```python
from build123d import *

# Parameters (mm, degrees)
SKETCH_1_W                  = 300
SKETCH_1_H                  = 30
EXTRUDE_1_DEPTH             = 5
CHAMFER_1_SIZE              = 1
HOLE_WIZARD_M3_1_D          = 3.2
M3X0_5_1_D                  = 2.5
M4X0_7_1_D                  = 3.3
M4X0_7_2_D                  = 3.3
PATTERN_LINEAR_1_COUNT      = 6
PATTERN_LINEAR_1_PITCH      = 25
PATTERN_LINEAR_1_COL_COUNT  = 7
PATTERN_LINEAR_1_COL_PITCH  = 25
EXTRUDE_3_DEPTH             = 5
SKETCH_13_R                 = 6.1
CUT_EXTRUDE_2_DEPTH         = 161.542829177
HOLE_WIZARD_M2_1_D          = 2.2
M4X0_7_3_D                  = 3.3
HOLE_WIZARD_M4_1_D          = 4.3
M3X0_5_2_D                  = 2.5
CUT_EXTRUDE_3_DEPTH         = 161.542829177
CUT_EXTRUDE_3_DEPTH_BACK    = 161.542829177
SKETCH_25_W                 = 15
SKETCH_25_H                 = 5
FILLET_1_R                  = 1
SKETCH_26_W                 = 30
SKETCH_26_H                 = 5
EXTRUDE_4_DEPTH             = 30
SKETCH_27_R                 = 1.65
CUT_EXTRUDE_4_DEPTH         = 174.476223155
PATTERN_LINEAR_2_COUNT      = 2
PATTERN_LINEAR_2_PITCH      = 20
PATTERN_LINEAR_2_COUNT_DIR2 = 3
PATTERN_LINEAR_2_PITCH_DIR2 = 10
FILLET_2_R                  = 5
HOLE_WIZARD_M3_2_D          = 3.2


with BuildPart() as part:
    # 草圖1 → 填料-伸長1 (new body)
    with BuildSketch(Plane.XY):
        Rectangle(SKETCH_1_W, SKETCH_1_H)
    extrude(amount=EXTRUDE_1_DEPTH)

    # 導角1
    chamfer_1_edges = [part.edges().sort_by_distance(p)[0] for p in [
        (150, -15, 2.5),
        (-150, -15, 2.5),
        (-150, 15, 2.5),
        (150, 15, 2.5),
    ]]
    chamfer(chamfer_1_edges, length=CHAMFER_1_SIZE)

    # M3 餘隙孔1 (through all)
    with Locations(Plane.XY.offset(5)):
        with Locations((20, -10), (20, 10), (0, -10), (0, 10)):
            Hole(HOLE_WIZARD_M3_1_D / 2)

    # M3x0.5 螺紋孔1 (through all)
    with Locations(Plane.XY.offset(5)):
        with Locations((-12.5, 0)):
            m3x0_5_1 = Hole(M3X0_5_1_D / 2)

    # M4x0.7 螺紋孔1 (through all)
    with Locations(Plane.XY.offset(5)):
        with Locations((100, 10), (70, -10), (70, 10), (100, -10), (85, 10), (85, -10)):
            Hole(M4X0_7_1_D / 2)

    # M4x0.7 螺紋孔2 (through all)
    with Locations(Plane.XY.offset(5)):
        with Locations((-126, 10), (-126, -10)):
            m4x0_7_2 = Hole(M4X0_7_2_D / 2)

    # 直線複製排列1: M3x0.5 螺紋孔1 ×6
    with Locations(*[(-i * PATTERN_LINEAR_1_PITCH, 0, 0) for i in range(1, PATTERN_LINEAR_1_COUNT)]):
        add(m3x0_5_1, mode=Mode.SUBTRACT)

    # 直線複製排列1 col: M3x0.5 螺紋孔1 ×7
    with Locations(*[(i * PATTERN_LINEAR_1_COL_PITCH, 0, 0) for i in range(1, PATTERN_LINEAR_1_COL_COUNT)]):
        add(m3x0_5_1, mode=Mode.SUBTRACT)

    # 鏡射1: M4x0.7 螺紋孔2 across plane
    add(m4x0_7_2.mirror(Plane(origin=(0, 0, 0), x_dir=(0, 0, 1), z_dir=(1, 0, 0))), mode=Mode.SUBTRACT)

    # 草圖16 → 填料-伸長3 (add, through all)
    with BuildSketch(Plane.XY):
        with BuildLine():
            Line((-20, 15), (64, 15))
            Line((64, 15), (64, 57))
            Line((64, 57), (0, 57))
            ThreePointArc((0, 57), (-14.142135624, 51.142135624), (-20, 37))
            Line((-20, 37), (-20, 15))
        make_face()
    extrude(amount=EXTRUDE_3_DEPTH)

    # 草圖13 → 除料-伸長2 (cut, through all)
    with BuildSketch(Plane.XY):
        with Locations(Location((44, 24.8, 0), (0, 0, 180))):
            Circle(SKETCH_13_R)
    extrude(amount=CUT_EXTRUDE_2_DEPTH, mode=Mode.SUBTRACT)

    # M2 餘隙孔1 (through all)
    with Locations(Plane.XY.offset(5)):
        with Locations((39, 24.8), (49, 24.8)):
            Hole(HOLE_WIZARD_M2_1_D / 2)

    # M4x0.7 螺紋孔3 (through all)
    with Locations(Plane.XY.offset(5)):
        with Locations((15, 22), (-15, 22)):
            Hole(M4X0_7_3_D / 2)

    # M4 餘隙孔1 (through all)
    with Locations(Plane.XY.offset(5)):
        with Locations((-26, -10), (-26, 10), (-50, -10), (-50, 10)):
            Hole(HOLE_WIZARD_M4_1_D / 2)

    # M3x0.5 螺紋孔2 (through all)
    with Locations(Plane.XY.offset(5)):
        with Locations((33, 53), (33, 45)):
            Hole(M3X0_5_2_D / 2)

    # 草圖25 → 除料-伸長3 (cut, two sides: drawn at the far end of the back side and taken through both)
    with BuildSketch(Plane.XY.offset(5).offset(-CUT_EXTRUDE_3_DEPTH_BACK)):
        with Locations((33, 38.5)):
            Rectangle(SKETCH_25_W, SKETCH_25_H)
    extrude(amount=CUT_EXTRUDE_3_DEPTH + CUT_EXTRUDE_3_DEPTH_BACK, mode=Mode.SUBTRACT)

    # 圓角1
    fillet_1_edges = [part.edges().sort_by_distance(p)[0] for p in [
        (40.5, 41, 2.5),
        (40.5, 36, 2.5),
        (25.5, 36, 2.5),
        (25.5, 41, 2.5),
    ]]
    fillet(fillet_1_edges, radius=FILLET_1_R)

    # 草圖26 → 填料-伸長4 (add)
    with BuildSketch(Plane(origin=(0, 57, 0), x_dir=(1, 0, 0), z_dir=(0, 1, 0))):
        with Locations((35, -2.5)):
            Rectangle(SKETCH_26_W, SKETCH_26_H)
    extrude(amount=EXTRUDE_4_DEPTH)

    # 草圖27 → 除料-伸長4 (cut, through all)
    with BuildSketch(Plane.XY.offset(5)):
        with Locations((25, 82)):
            Circle(SKETCH_27_R)
    cut_extrude_4 = extrude(amount=-CUT_EXTRUDE_4_DEPTH, mode=Mode.SUBTRACT)

    # 直線複製排列2: Cut-Extrude 4 2 × 3
    with Locations(*[(i * PATTERN_LINEAR_2_PITCH, -j * PATTERN_LINEAR_2_PITCH_DIR2, 0) for i in range(PATTERN_LINEAR_2_COUNT) for j in range(PATTERN_LINEAR_2_COUNT_DIR2) if (i, j) != (0, 0)]):
        add(cut_extrude_4, mode=Mode.SUBTRACT)

    # 圓角2
    fillet_2_edges = [part.edges().sort_by_distance(p)[0] for p in [
        (50, 87, 2.5),
        (20, 87, 2.5),
    ]]
    fillet(fillet_2_edges, radius=FILLET_2_R)

    # M3 餘隙孔2 (through all)
    with Locations(Plane.XY.offset(5)):
        with Locations((36.25, 4.376606241), (28.5, 17.8), (59.5, 17.8), (36.25, 31.223393759), (51.75, 4.376606241), (51.75, 31.223393759)):
            Hole(HOLE_WIZARD_M3_2_D / 2)


solid = part.part
```
Can you work these out from the model? Positions are in its coordinate system, mm. A direction names the side the tool comes from. Give positions to 0.01 mm unless a question says otherwise; leave off trailing zeros. Write each loop counter-clockwise with the first axis right and the second up, starting at its lowest first coordinate (ties: lowest second). Pieces come first, ordered by that corner, then holes. Notation, with made-up numbers: (41.25, -36.5) -> (72.25, -36.5) arc R13 cw to (72.25, -25.5) -> close; hole circle Ø11 at (33, -16). An arc over 180 degrees is marked (long way). One line per item, written item: value.
Q1. We'd pull the mould along X, two halves only. Please class faces 1 (the face through (-2, 14, 5)), 2 (the face through (38.18, 22.97, 2.46)), 3 (the face through (20, 69, 3)): +X half, -X half, draft (parallel to the pull), parting line (faces both ways), or undercut.
Results found:
face 1: draft
face 2: undercut
face 3: -X half
Q2. Imagine slicing it at A-A on x = -73. Please give me the cut outline in (y, z), and give its area (3 significant figures).
Results found:
outline: (-15, 0) -> (15, 0) -> (15, 5) -> (-15, 5) -> close
area: 150 mm^2
Q3. For P1, Ø3.5, axis at x = 36.25, y = 31.22, coming from the +Z side; P2, Ø2.5, axis at x = 55, z = 1.5, coming from the +Y side; P3, Ø1.5, axis at x = 85.5, z = 3.5, coming from the +Y side, each with a flat end and sliding along its axis, tell me the tip position at first contact or that it passes through.
Results found:
P1: stops at z = 5
P2: stops at y = 57
P3: stops at y = 15
Q4. Imagine slicing it at B-B on z = 3.25. Give the number of separate pieces and of enclosed holes in the cut face, and give its area (3 significant figures).
Results found:
separate pieces: 1
enclosed holes: 48
area: 12,800 mm^2
Q5. Which directions (+Z, -Z, +X, -X, +Y, -Y) give clear straight access to the entire face, cutting with the end or side of a thin tool? Please do faces 4 (the face through (10, 57, 2)), 5 (the face through (57, 57, 2)), 6 (the face through (33, 41, 2)), 7 (the face through (-2, 14, 0)).
Results found:
face 4: +Z, -Z, -X, +Y
face 5: +Z, -Z, +X, +Y
face 6: +Z, -Z
face 7: -Z, +X, -X, +Y, -Y
Q6. Please list where these lines run through material, in increasing order: line 1 (Y direction, x = -26, z = 3.3); line 2 (Y direction, x = 85, z = 2.6); line 3 (Y direction, x = 33, z = 3.6). Write a range as [from, to].
Results found:
line 1: y = [-15, -12.15], [-7.85, 7.85], [12.15, 15]
line 2: y = [-15, -11.65], [-8.35, 8.35], [11.65, 15]
line 3: y = [-15, 36], [41, 43.75], [46.25, 51.75], [54.25, 87]
